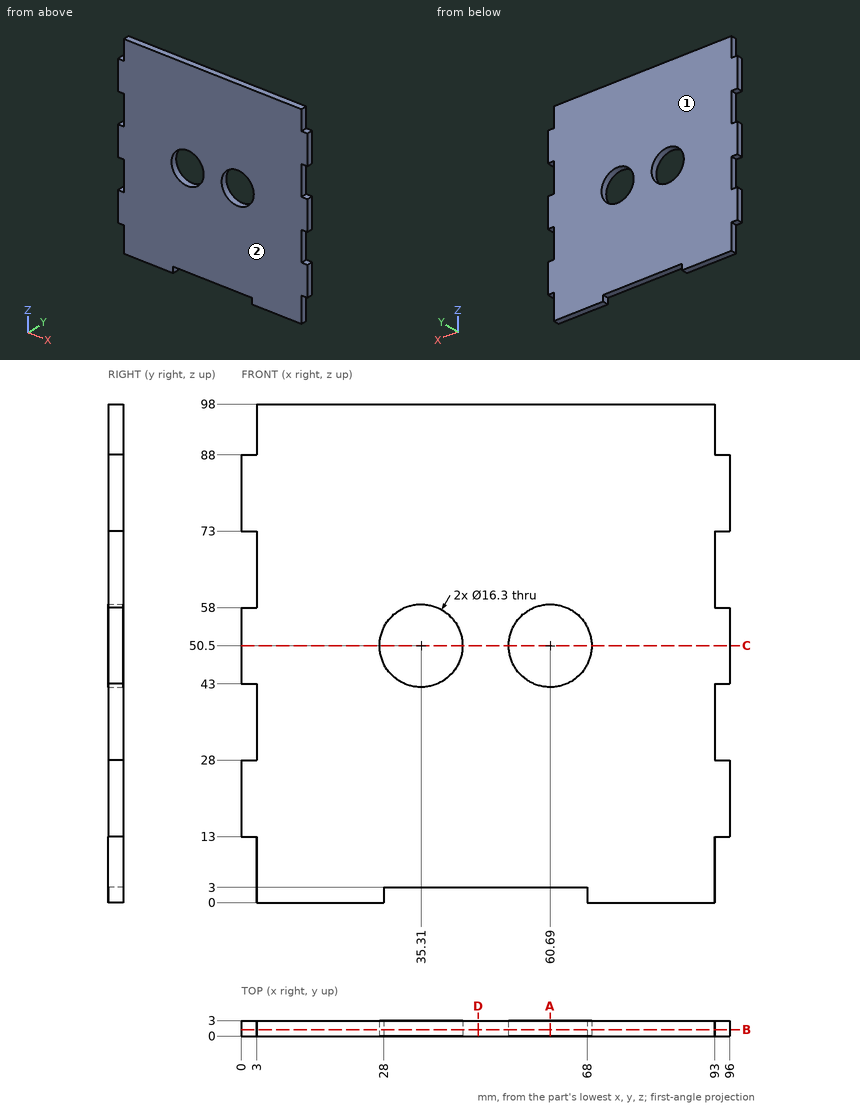
Geometry: see drawing. Coordinates: mm, zero at the bounding-box minimum. Round coordinates to 2 decimals unless told otherwise and drop trailing zeros. Order: outer loops, then holes, each group sorted by start corner. A loop starts at its lowest first (then second) coordinate and runs counter-clockwise, first axis right, second up. Notation, with made-up numbers: (36, 23.25) - (62, 23.25) arc R8 ccw to (62, 31.25) - close; hole circle Ø9 at (44.25, 60.25). An arc over 180 degrees is marked (long way). Use a Markdown table: item, result. Add a question column.
1. Section query D-D (x = 46.5). Return the cut outline in (y, z), then the cut area to 3 significant figures.
2. Section query C-C (z = 50.5). Return the cut outline in (x, y).
3. Line query: probe 1 along X at (y, z) = (1.6, 50.5); probe 2 along Z at (x, y) = (35.31, 0.85); probe 3 along X at (y, z) = (2, 54). Output: solid intervals per line, ascending.
4. Section query B-B (y = 1.25). Give the number of separate pieces and of enclosed holes in the cut face, then the cut area to 3 significant figures.
5. Mould query, pull axis Y, two halves, no side actions, for the marked faces 1 and 2. Classes: +Y half, -Y half, draft (parallel to the pull), parting line (faces both ways), or undercut.
6. Section query A-A (x = 60.69). Return the cut outline in (y, z).
7. First-contact query: pin 1 (1 mm diameter, centred on x = 42.5, z = 60, fed in from -Y); pin 2 (10 mm diameter, centred on x = 35.31, z = 50.5, fed in from -Y); pin 3 (0.9 mm diameter, centred on x = 2, y = 1.5, fed in from -Z). Flat tips, straight axial feed; report the tip coordinate or a pass-through.
Derived:
| question | item | result |
|---|---|---|
| 1 | outline | (0, 3) - (3, 3) - (3, 98) - (0, 98) - close |
| 1 | area | 285 mm2 |
| 2 | outline | (0, 0) - (27.16, 0) - (27.16, 3) - (0, 3) - close; (43.46, 0) - (52.54, 0) - (52.54, 3) - (43.46, 3) - close; (68.84, 0) - (96, 0) - (96, 3) - (68.84, 3) - close |
| 3 | probe 1 | 0 to 27.16, 43.46 to 52.54, 68.84 to 96 |
| 3 | probe 2 | 3 to 42.35, 58.65 to 98 |
| 3 | probe 3 | 0 to 27.95, 42.67 to 53.33, 68.05 to 96 |
| 4 | separate pieces | 1 |
| 4 | enclosed holes | 2 |
| 4 | area | 8,550 mm2 |
| 5 | face 1 | +Y half |
| 5 | face 2 | -Y half |
| 6 | outline | (0, 3) - (3, 3) - (3, 42.35) - (0, 42.35) - close; (0, 58.65) - (3, 58.65) - (3, 98) - (0, 98) - close |
| 7 | pin 1 | y = 0 |
| 7 | pin 2 | through |
| 7 | pin 3 | z = 13 |
